Geometry: final body of the model. Coordinates: model frame, mm. Round coordinates to 2 decimals unless told otherwise and drop trailing zeros. Write each loop counter-clockwise with the first axis right and the second up, starting at its lowest first coordinate (ties: lowest second). Pieces come first, ordered by that corner, then holes. Notation, with made-up numbers: (57, 67) - (100, 67) arc R10 cw to (100, 82) - close; hole circle Ø7 at (52, 65.25). An arc over 180 degrees is marked (long way). Write each question's results on one line, items separated by ' | '.
from build123d import *

# Parameters (mm, degrees)
F1_DEPTH = 3
F2_D     = 3.4


with BuildPart() as f1:
    # F0 (on Top) → F1 (new body)
    with BuildSketch(Plane.XY):
        with BuildLine():
            ThreePointArc((-55.6590960491, 92.5530389939), (-51.154476682, 95.1168729269), (-46.5320369414, 97.4616311072))
            Line((-46.5320369414, 97.4616311072), (-59.0267505646, 123.6318839045))
            ThreePointArc((-59.0267505646, 123.6318839045), (-64.8904009762, 120.6575147314), (-70.6045940623, 117.4052439089))
            ThreePointArc((-70.6045940623, 117.4052439089), (-87.6662762423, 105.278791833), (-102.6814380892, 90.6946650688))
            ThreePointArc((-102.6814380892, 90.6946650688), (-106.9145490542, 85.6637566334), (-110.9014115399, 80.4355451181))
            Line((-110.9014115399, 80.4355451181), (-87.4259302651, 63.4090428669))
            ThreePointArc((-87.4259302651, 63.4090428669), (-84.2830021741, 67.5305526745), (-80.9459511944, 71.4965242878))
            ThreePointArc((-80.9459511944, 71.4965242878), (-69.1091812713, 82.9935001311), (-55.6590960491, 92.5530389939))
        make_face()
    extrude(amount=F1_DEPTH)

    # F2 (through all)
    with Locations(Plane(origin=(0, 0, 0), x_dir=(1, 0, 0), z_dir=(0, 0, -1))):
        with Locations((-98.9339403487, -87.3846407962), (-84.6934489349, -74.8065485604), (-58.2359060514, -96.8379019102), (-68.02778406, -113.1203809925)):
            Hole(F2_D / 2)


solid = f1.part
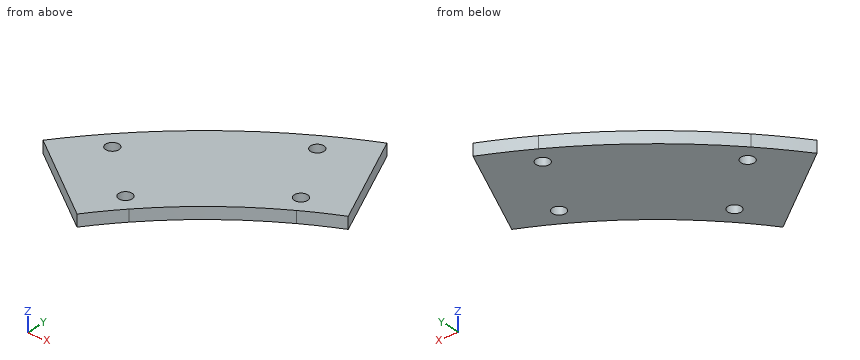
Q1. Section query A-A, the plane x = -85. Return loops of the section in (y, z), plus the area to 3 significant figures.
Answer block:
outline: (66.63, 0) - (73.13, 0) - (73.13, 3) - (66.63, 3) - close; (76.48, 0) - (107.44, 0) - (107.44, 3) - (76.48, 3) - close | area: 112 mm2
Q2. Section query D-D, the plane x = -53. Return loops of the section in (y, z), plus the area to 3 significant figures.
Answer block:
outline: (94.1, 0) - (111.01, 0) - (111.01, 3) - (94.1, 3) - close | area: 50.7 mm2
Q3. Section query C-C, the plane y = 78. Return loops of the section in (x, z).
Answer block:
outline: (-107.54, 0) - (-74.7, 0) - (-74.7, 3) - (-107.54, 3) - close
Q4. Pin query (flat end, axial travel): pin 1 (3 mm diameter, centred on x = -68.03, y = 113.12, fed in from -Z); pin 2 (1 mm diameter, centred on x = -79, z = 2.5, fed in from -Y); pin 3 (1.5 mm diameter, centred on x = -69, z = 2, fed in from +Y); pin 4 (1 mm diameter, centred on y = 110.5, z = 2.5, fed in from +X). Return the tip coordinate at first contact, or that it passes through.
Answer block:
pin 1: through | pin 2: y = 73.1 | pin 3: y = 118.79 | pin 4: x = -52.52
Q5. Section query B-B, the plane z = 0.5. Return loops of the section in (x, y), plus the area to 3 significant figures.
Answer block:
outline: (-110.9, 80.44) - (-87.43, 63.41) arc R108 cw to (-46.53, 97.46) - (-59.03, 123.63) arc R137 ccw to start; hole circle Ø3.4 at (-98.93, 87.38); hole circle Ø3.4 at (-84.69, 74.81); hole circle Ø3.4 at (-68.03, 113.12); hole circle Ø3.4 at (-58.24, 96.84) | area: 1,730 mm2
Q6. Ray query, line 1 along Y through (x, z) = (-99, 0.15); line 2 along X through (y, z) = (96, 1.7); line 3 along X through (y, z) = (113, 0.75). Return the intervals inside material, ascending.
Answer block:
line 1: 71.8 to 85.69, 89.08 to 94.7 | line 2: -97.74 to -59.72, -56.76 to -49.48 | line 3: -77.46 to -69.72, -66.33 to -53.95
